Here's how the part is built. I have some questions about the finished solid (model axes, mm). A direction names the side the tool comes from. Coordinates: 2 decimals unless noted, no trailing zeros. Order: outer loops, then holes, each group sorted by start corner. A loop starts at its lowest first (then second) coordinate and runs counter-clockwise, first axis right, second up. Notation, with made-up numbers: (-16, 66) - (-7, 66) arc R15 cw to (-7, 83) - close; hole circle Ø2 at (87.5, 19.5). An arc over 180 degrees is marked (long way). Answer as CSV lines item,"result". Start each with the question number.
Q1. I need wall thicknesses on line 1 (X direction, y = 77.5, z = -24); line 2 (Z direction, x = 42, y = 71.5); line 3 (Y direction, x = -50, z = 37.5). Which ranges of each line are inside material? Lowest first, please.
Q2. Suppose I cut it at D-D (y = 46.5). Please give me the cut outline in (x, z).
Q3. Thinking about a two-plate mould opening in Y: for faces 4 (the face through (-89, 12, 0)), 5 (the face through (88.986, 10.601, -31.908)), 6 (the face through (-4.91, 88.52, 35.95)), 7 (the face through (-41, 90, -1)), which applies, released by +Y, released by -Y, zero draft, split by the parting line, or undercut?
Q4. Suppose I cut it at A-A (x = 51). Please give me the cut outline in (y, z), then the cut area to 3 significant figures.
Q5. Suppose I cut it at C-C (z = 5.5). Please give me the cut outline in (x, y), then the cut area to 3 significant figures.
Q6. Suppose I cut it at B-B (x = -60). Please give me the cut outline in (y, z).
Q7. For pin 1 Ø5 at (x, z) = (-60, -22.95) entering from -Y; pin 2 Ø2.5 at (y, z) = (10, -30) entering from +X; pin 3 Ø2.5 at (y, z) = (10, -20) entering from -X, each with a flat end and sliding along its axis, tell me the tip position at first contact or that it passes through.
Q8. For faces 1 (the face through (84.99, 44.37, -45.15)), 2 (the face through (88.986, 10.601, 28.092)), 3 (the face through (89, 8, -10)), which set-ups out of +Z, -Z, +X, -X, +Y, -Y let a thin tool reach every point of the face, with its end or its side?
from build123d import *

# Parameters (mm, degrees)
Y_KSEKLIK_EKSTR_ZYON1_DEPTH = 90
IZIM2_W                     = 75
IZIM2_H                     = 100
Y_KSEKLIK_EKSTR_ZYON2_DEPTH = 3
IZIM3_R                     = 2
KES_EKSTR_ZYON1_DEPTH       = 10
IZIM4_R                     = 2
KES_EKSTR_ZYON2_DEPTH       = 10
KES_EKSTR_ZYON3_START       = -10
IZIM5_R                     = 2
KES_EKSTR_ZYON3_DEPTH       = 10


with BuildPart() as part:
    # Çizim1 → Yükseklik-Ekstrüzyon1 (new body)
    with BuildSketch(Plane(origin=(0, 0, 0), x_dir=(1, 0, 0), z_dir=(0, 1, 0))):
        with BuildLine():
            Line((-70, -50), (80, -50))
            ThreePointArc((80, -50), (87.071067812, -47.071067812), (90, -40))
            Line((90, -40), (90, 40))
            ThreePointArc((90, 40), (87.071067812, 47.071067812), (80, 50))
            Line((80, 50), (-70, 50))
            ThreePointArc((-70, 50), (-84.142135624, 44.142135624), (-90, 30))
            Line((-90, 30), (-90, -30))
            ThreePointArc((-90, -30), (-84.142135624, -44.142135624), (-70, -50))
        make_face()
        with BuildLine():
            Line((0, 48), (78, 48))
            ThreePointArc((78, 48), (85.071067812, 45.071067812), (88, 38))
            Line((88, 38), (88, 0))
            Line((88, 0), (88, -38))
            ThreePointArc((88, -38), (85.071067812, -45.071067812), (78, -48))
            Line((78, -48), (-68, -48))
            ThreePointArc((-68, -48), (-82.142135624, -42.142135624), (-88, -28))
            Line((-88, -28), (-88, 28))
            ThreePointArc((-88, 28), (-82.142135624, 42.142135624), (-68, 48))
            Line((-68, 48), (0, 48))
        make_face(mode=Mode.SUBTRACT)
    extrude(amount=Y_KSEKLIK_EKSTR_ZYON1_DEPTH)

    # Çizim2 → Yükseklik-Ekstrüzyon2 (add)
    with BuildSketch(Plane(origin=(0, 90, 0), x_dir=(1, 0, 0), z_dir=(0, 1, 0))):
        with Locations((-32.5, 0)):
            Rectangle(IZIM2_W, IZIM2_H)
    extrude(amount=-Y_KSEKLIK_EKSTR_ZYON2_DEPTH)

    # Çizim3 → Kes-Ekstrüzyon1 (cut)
    with BuildSketch(Plane.ZY.offset(90)):
        with Locations((-20, 10)):
            Circle(IZIM3_R)
        with Locations((-10, 10)):
            Circle(IZIM3_R)
        with Locations((0, 10)):
            Circle(IZIM3_R)
        with Locations((10, 10)):
            Circle(IZIM3_R)
        with Locations((20, 10)):
            Circle(IZIM3_R)
    extrude(amount=-KES_EKSTR_ZYON1_DEPTH, mode=Mode.SUBTRACT)

    # Çizim4 → Kes-Ekstrüzyon2 (cut)
    with BuildSketch(Plane(origin=(0, 90, 0), x_dir=(1, 0, 0), z_dir=(0, 1, 0))):
        with Locations(Location((-60, 37.949874371, 0), (0, 0, 270))):
            Circle(IZIM4_R)
        with Locations(Location((-45, 37.949874371, 0), (0, 0, 270))):
            Circle(IZIM4_R)
        with Locations(Location((-60, 22.949874371, 0), (0, 0, 270))):
            Circle(IZIM4_R)
        with Locations(Location((-5, 22.949874371, 0), (0, 0, 90))):
            Circle(IZIM4_R)
        with Locations(Location((-20, 37.949874371, 0), (0, 0, 90))):
            Circle(IZIM4_R)
        with Locations(Location((-5, 37.949874371, 0), (0, 0, 90))):
            Circle(IZIM4_R)
        with Locations(Location((-5, -37.949874371, 0), (0, 0, 270))):
            Circle(IZIM4_R)
        with Locations(Location((-20, -37.949874371, 0), (0, 0, 270))):
            Circle(IZIM4_R)
        with Locations(Location((-5, -22.949874371, 0), (0, 0, 270))):
            Circle(IZIM4_R)
        with Locations(Location((-60, -22.949874371, 0), (0, 0, 90))):
            Circle(IZIM4_R)
        with Locations(Location((-45, -37.949874371, 0), (0, 0, 90))):
            Circle(IZIM4_R)
        with Locations(Location((-60, -37.949874371, 0), (0, 0, 90))):
            Circle(IZIM4_R)
    extrude(amount=-KES_EKSTR_ZYON2_DEPTH, mode=Mode.SUBTRACT)

    # Çizim5 → Kes-Ekstrüzyon3 (cut)
    with BuildSketch(Plane(origin=(90, 0, 0), x_dir=(0, 0, -1), z_dir=(1, 0, 0)).offset(KES_EKSTR_ZYON3_START)):
        with Locations((-30, 10)):
            Circle(IZIM5_R)
        with Locations(Location((-10, 10, 0), (0, 0, 180))):
            Circle(IZIM5_R)
        with Locations(Location((10, 10, 0), (0, 0, 180))):
            Circle(IZIM5_R)
        with Locations((30, 10)):
            Circle(IZIM5_R)
    extrude(amount=KES_EKSTR_ZYON3_DEPTH, mode=Mode.SUBTRACT)


solid = part.part
Here are the results:
1,line 1,"x = -90 to -88, 88 to 90"
1,line 2,"z = -50 to -48, 48 to 50"
1,line 3,"y = 87 to 90"
2,outline,"(-90, -30) arc R20 ccw to (-70, -50) - (80, -50) arc R10 ccw to (90, -40) - (90, 40) arc R10 ccw to (80, 50) - (-70, 50) arc R20 ccw to (-90, 30) - close; hole (-88, -28) arc R20 ccw to (-68, -48) - (78, -48) arc R10 ccw to (88, -38) - (88, 38) arc R10 ccw to (78, 48) - (-68, 48) arc R20 ccw to (-88, 28) - close"
3,face 4,"undercut"
3,face 5,"undercut"
3,face 6,"zero draft"
3,face 7,"released by +Y"
4,outline,"(0, -50) - (90, -50) - (90, -48) - (0, -48) - close; (0, 48) - (90, 48) - (90, 50) - (0, 50) - close"
4,area,"360 mm²"
5,outline,"(-90, 0) - (-88, 0) - (-88, 90) - (-90, 90) - close; (-70, 87) - (5, 87) - (5, 90) - (-70, 90) - close; (88, 0) - (90, 0) - (90, 90) - (88, 90) - close"
5,area,"585 mm²"
6,outline,"(0, -50) - (90, -50) - (90, -39.95) - (87, -39.95) - (87, -48) - (0, -48) - close; (0, 48) - (87, 48) - (87, 39.95) - (90, 39.95) - (90, 50) - (0, 50) - close; (87, -35.95) - (90, -35.95) - (90, -24.95) - (87, -24.95) - close; (87, -20.95) - (90, -20.95) - (90, 20.95) - (87, 20.95) - close; (87, 24.95) - (90, 24.95) - (90, 35.95) - (87, 35.95) - close"
7,pin 1,"stops at y = 87"
7,pin 2,"stops at x = -87.73"
7,pin 3,"stops at x = 88"
8,face 1,"+Y, -Y"
8,face 2,"+X"
8,face 3,"+X, -X"
